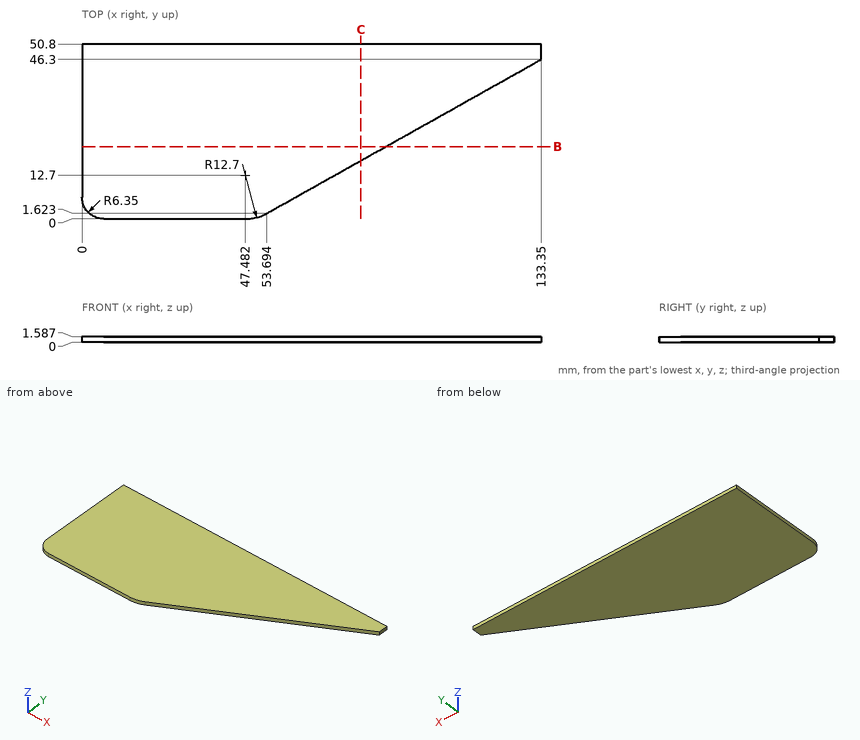
Geometry check sheet. Reference: drawing and pictorial views, mm from the part's lowest x, y, z. Give positions to 0.01 mm unless a question says otherwise; leave off trailing zeros. Order: outer loops, then holes, each group sorted by start corner. A loop starts at its lowest first (then second) coordinate and runs counter-clockwise, first axis right, second up. Notation, with made-up numbers: (76, 30.5) - (120, 30.5) arc R7 cw to (120, 42.5) - close; hole circle Ø1 at (84, 7.5). An arc over 180 degrees is marked (long way). Answer as CSV lines item,"result". Start each with the question number.
Item 1: Section check B-B, the plane y = 21. Record the boundary of the cut face in (x, z).
Item 2: Material ranges on L1, parallel to X at y = 42, z = 0.9 (1 decimal); L2, parallel to Y at x = 67, z = 0.5 (1 decimal); L3, parallel to X at y = 18.5, z = 0.6 (1 decimal), recorded low to high.
Item 3: Section check C-C, the plane x = 81. Record the boundary of the cut face in (y, z).
Filled in:
1,outline,"(0, 0) - (88.24, 0) - (88.24, 1.59) - (0, 1.59) - close"
2,L1,"0 to 125.7"
2,L2,"9.1 to 50.8"
2,L3,"0 to 83.8"
3,outline,"(16.94, 0) - (50.8, 0) - (50.8, 1.59) - (16.94, 1.59) - close"
